Study the drawing (mm; zero at the part's minimum x, y, z) and answer. A direction names the side the tool comes from. Round coordinates to 2 decimals unless told otherwise and drop trailing zeros. Write each loop counter-clockwise with the first axis right and the second up, starting at its lowest first coordinate (ties: lowest second). Pieces come first, ordered by that corner, then holes.
(1) A cutting plane is placed at C-C, the plane y = 4. Give the vertices of the cut face in (x, z) (1 decimal), and give its area (3 significant figures).
(2) For the marked faces 5, 6 and 7, determine the directions among +Z, -Z, +X, -X, +Y, -Y from which every point of the face is accessible in a straight line to the end or side of a thin tool.
(3) A cutting plane is placed at A-A, the plane z = 36.83. Give the vertices of the cut face in (x, y) (1 decimal), and give its area (3 significant figures).
(4) The mould has two halves that part along Z. Classify the marked faces 1, 2, 3 and 4: +Z half, -Z half, draft (parallel to the pull), parting line (faces both ways), or undercut.
(5) Find the intervals of material crossed by probe 1 along Z at (x, y) = (19, 2) (1 decimal); probe 2 along Y at (x, z) = (32, 43.5) (1 decimal); probe 3 along Z at (x, y) = (26, 19) (1 decimal), in increasing order.
(6) Each of these flat-tipped pins is pushed along its axis until it touches: pin 1 Ø1 at (y, z) = (28, 52) entering from +X (1 decimal); pin 2 Ø2.5 at (y, z) = (13, 52.5) entering from -X (1 decimal); pin 3 Ø4 at (x, z) = (33.34, 22.22) entering from +Y. Where does it stop, or does it pass through?
(7) A cutting plane is placed at B-B, the plane x = 19.05. Give the number of separate pieces and of enclosed holes in the cut face, and give its area (3 significant figures).
(8) A cutting plane is placed at D-D, the plane z = 29. Give the vertices of the cut face in (x, y) (1 decimal).
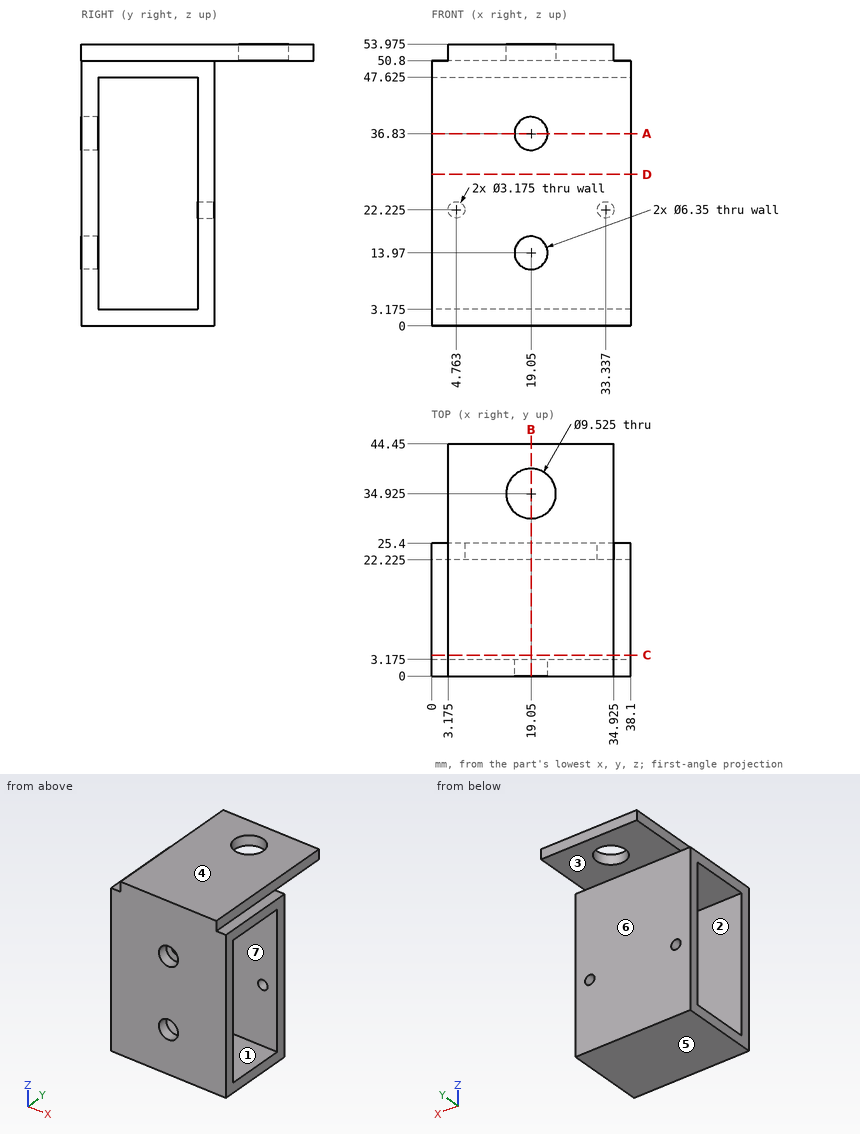
Solutions:
1. outline: (0, 0) - (38.1, 0) - (38.1, 3.2) - (0, 3.2) - close; (0, 47.6) - (38.1, 47.6) - (38.1, 50.8) - (34.9, 50.8) - (34.9, 54) - (3.2, 54) - (3.2, 50.8) - (0, 50.8) - close
1. area: 343 mm2
2. face 5: -Z, +X, -X, +Y, -Y
2. face 6: -Z, +X, -X, +Y
2. face 7: +X, -X
3. outline: (0, 0) - (15.9, 0) - (15.9, 3.2) - (0, 3.2) - close; (0, 22.2) - (38.1, 22.2) - (38.1, 25.4) - (0, 25.4) - close; (22.2, 0) - (38.1, 0) - (38.1, 3.2) - (22.2, 3.2) - close
3. area: 222 mm2
4. face 1: undercut
4. face 2: undercut
4. face 3: -Z half
4. face 4: +Z half
5. probe 1: z = 0 to 10.8, 17.1 to 33.7, 40 to 54
5. probe 2: y = 0 to 3.2, 22.2 to 25.4
5. probe 3: z = 0 to 3.2, 47.6 to 54
6. pin 1: stops at x = 34.9
6. pin 2: stops at x = 3.2
6. pin 3: stops at y = 25.4
7. separate pieces: 3
7. enclosed holes: 0
7. area: 514 mm2
8. outline: (0, 0) - (38.1, 0) - (38.1, 3.2) - (0, 3.2) - close; (0, 22.2) - (38.1, 22.2) - (38.1, 25.4) - (0, 25.4) - close
